Build history of the part. All positions in model axes, mm. A direction names the side the tool comes from. Round coordinates to 2 decimals unless told otherwise and drop trailing zeros. Write each loop counter-clockwise with the first axis right and the second up, starting at its lowest first coordinate (ties: lowest second). Pieces come first, ordered by that corner, then holes. Notation, with made-up numbers: (53, -14) - (85, -14) arc R9 ccw to (85, -2) - close; hole circle Ø4 at (-21, -33). An arc over 180 degrees is marked (long way). Write each question's results on one line, items separated by ' | '.
from build123d import *

# Parameters (mm, degrees)
SKETCH1_W           = 44.15
SKETCH1_H           = 25.908
BOSS_EXTRUDE1_DEPTH = 17.018
SKETCH2_R           = 3.556
BOSS_EXTRUDE2_DEPTH = 4.7
SKETCH3_R           = 2.438606829
CUT_EXTRUDE1_DEPTH  = 3.81


with BuildPart() as part:
    # Sketch1 → Boss-Extrude1 (new body)
    with BuildSketch(Plane.XY):
        with Locations((22.075, 12.954)):
            Rectangle(SKETCH1_W, SKETCH1_H)
    extrude(amount=BOSS_EXTRUDE1_DEPTH)

    # Sketch2 → Boss-Extrude2 (add)
    with BuildSketch(Plane.ZY):
        with Locations(Location((8.509, 6.602690832, 0), (0, 0, 180))):
            Circle(SKETCH2_R)
        Polygon((14.027892204, 20.883427677), (10.795, 24.116319881), (6.223, 24.116319881), (2.990107796, 20.883427677), (2.990107796, 16.311427677), (6.223, 13.078535474), (10.795, 13.078535474), (14.027892204, 16.311427677), align=None)
    extrude(amount=BOSS_EXTRUDE2_DEPTH)

    # Sketch3 → Cut-Extrude1 (cut)
    with BuildSketch(Plane.ZY.offset(4.7)):
        with Locations((8.509, 6.602690832)):
            Circle(SKETCH3_R)
        Polygon((12.568856448, 20.376314243), (10.129301757, 22.729112808), (6.740596271, 22.667766962), (4.387797706, 20.228212271), (4.449143552, 16.839506785), (6.888698243, 14.48670822), (10.277403729, 14.548054066), (12.630202294, 16.987608757), align=None)
    extrude(amount=-CUT_EXTRUDE1_DEPTH, mode=Mode.SUBTRACT)


solid = part.part
(1) Tool access for faces 4 (the flat face through (-2.822, 21.465, 5.581)), 5 (the flat face through (-2, 24.116, 9)), 6 (the flat face through (-2, 13.079, 8)), 7 (the flat face through (-2.32, 22.48, 12.43)), 8 (the flat face through (-2.317, 14.672, 12.389)): list every direction of +Z, -Z, +X, -X, +Y, -Y with a clear straight run to the whole face (end or side of a thin tool).
Worked answers:
face 4: -X | face 5: +Z, -Z, -X, +Y | face 6: +Z, -Z, -X | face 7: +Z, -X, +Y | face 8: +Z, -X
(2) Slice it at A-A, the plane y = 13.75. Write the cut outline in (x, z), and give its area (3 significant figures).
Worked answers:
outline: (-4.7, 5.55) - (0, 5.55) - (0, 0) - (44.15, 0) - (44.15, 17.02) - (0, 17.02) - (0, 11.47) - (-4.7, 11.47) - close | area: 779 mm2
(3) Slice it at C-C, the plane y = 5. Write the cut outline in (x, z).
Worked answers:
outline: (-4.7, 5.33) - (0, 5.33) - (0, 0) - (44.15, 0) - (44.15, 17.02) - (0, 17.02) - (0, 11.68) - (-4.7, 11.68) - (-4.7, 10.35) - (-0.89, 10.35) - (-0.89, 6.67) - (-4.7, 6.67) - close
(4) Slice it at B-B, the plane z = 9. Write the cut outline in (x, y), and give its area (3 significant figures).
Worked answers:
outline: (-4.7, 3.08) - (0, 3.08) - (0, 0) - (44.15, 0) - (44.15, 25.91) - (0, 25.91) - (0, 24.12) - (-4.7, 24.12) - (-4.7, 22.71) - (-0.89, 22.71) - (-0.89, 14.52) - (-4.7, 14.52) - (-4.7, 13.08) - (0, 13.08) - (0, 10.12) - (-4.7, 10.12) - (-4.7, 8.99) - (-0.89, 8.99) - (-0.89, 4.21) - (-4.7, 4.21) - close | area: 1,180 mm2
(5) Flat gauge pins, fed straight in: pin 1 Ø3.5 at (x, y) = (-3.5, 19.5) entering from +Z; pin 2 Ø3.5 at (x, z) = (-2, 7.5) entering from -Y; pin 3 Ø5 at (x, z) = (-3.5, 8.5) entering from +Y. Where does each tip first touch, or does it go through?
Worked answers:
pin 1: stops at z = 14.03 | pin 2: stops at y = 3.05 | pin 3: stops at y = 24.12
(6) Two-plate mould, pull along Y, no slides. Class faces 1 (the flat face through (-0.89, 19, 8)), 2 (the flat face through (-2, 19, 14.028)), 3 (the flat face through (22, 25.908, 8)): released by +Y, released by -Y, zero draft, split by the parting line, or undercut.
Worked answers:
face 1: undercut | face 2: zero draft | face 3: released by +Y
(7) Drill centre lines: probe 1 along X at (y, z) = (2, 8); probe 2 along X at (y, z) = (21, 10); probe 3 along Z at (x, y) = (-1.5, 8.75). Where is each one in solid material? Low to high. Write a range as [from, to].
Worked answers:
probe 1: x = [0, 44.15] | probe 2: x = [-0.89, 44.15] | probe 3: z = [5.67, 7.35], [9.66, 11.34]
(8) Slice it at D-D, the plane z = 14.5. Write the cut outline in (x, y).
Worked answers:
outline: (0, 0) - (44.15, 0) - (44.15, 25.91) - (0, 25.91) - close
